```python
from build123d import *

# Parameters (mm, degrees)
BOSS_EXTRUDE1_DEPTH = 3
SKETCH2_R           = 2.125
SKETCH2_R_2         = 1.375
CUT_EXTRUDE1_DEPTH  = 57.401986652


with BuildPart() as part:
    # Sketch1 → Boss-Extrude1 (new body)
    with BuildSketch(Plane(origin=(0, 0, 0), x_dir=(1, 0, 0), z_dir=(0, 1, 0))):
        with BuildLine():
            Line((-31.972318339, 0), (13.027681661, 0))
            ThreePointArc((13.027681661, 0), (28.332991201, -15.30530954), (13.027681661, -30.61061908))
            Line((13.027681661, -30.61061908), (-31.972318339, -30.61061908))
            ThreePointArc((-31.972318339, -30.61061908), (-47.277627879, -15.30530954), (-31.972318339, 0))
        make_face()
    extrude(amount=BOSS_EXTRUDE1_DEPTH)

    # Sketch2 → Cut-Extrude1 (cut, through all)
    with BuildSketch(Plane(origin=(0, 3, 0), x_dir=(1, 0, 0), z_dir=(0, 1, 0))):
        with Locations(Location((-31.972318339, -15.30530954, 0), (0, 0, 270))):
            Circle(SKETCH2_R)
        with Locations(Location((-31.972318339, -5.30530954, 0), (0, 0, 270))):
            Circle(SKETCH2_R_2)
        with Locations(Location((-31.972318339, -25.30530954, 0), (0, 0, 90))):
            Circle(SKETCH2_R_2)
        with Locations(Location((13.027681661, -5.30530954, 0), (0, 0, 90))):
            Circle(SKETCH2_R_2)
        with Locations(Location((13.027681661, -15.30530954, 0), (0, 0, 90))):
            Circle(SKETCH2_R)
        with Locations(Location((13.027681661, -25.30530954, 0), (0, 0, 270))):
            Circle(SKETCH2_R_2)
    extrude(amount=-CUT_EXTRUDE1_DEPTH, mode=Mode.SUBTRACT)


solid = part.part
```
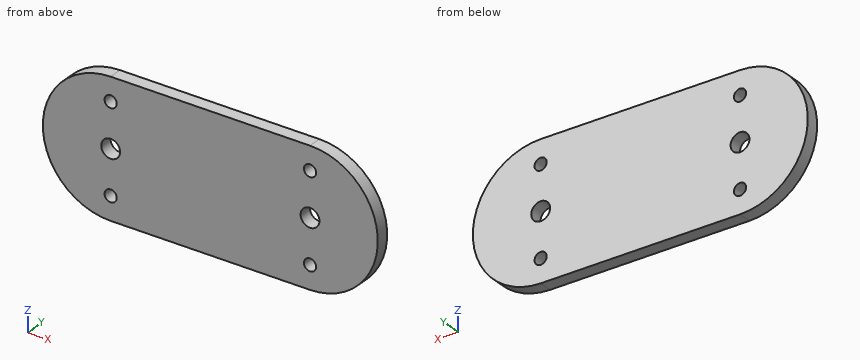
Verification items for the finished model (mm, model axes). Coordinates: 2 decimals unless noted, no trailing zeros. Loops run counter-clockwise (first coordinate to the right, second up) from the corner with the lowest first, then second, coordinate; pieces in that order, holes last. Notation, with made-up numbers: (12.25, 9.25) -> (30.25, 9.25) arc R34 ccw to (30.25, 46.25) -> close; hole circle Ø11 at (0, 11.25). An arc over 180 degrees is marked (long way). Put each result on its own line as item: value.
1. Section check B-B, the plane z = 14. Record the boundary of the cut face in (x, y).
Result set:
outline: (-47.22, 0) -> (-33.65, 0) -> (-33.65, 3) -> (-47.22, 3) -> close; (-30.3, 0) -> (11.35, 0) -> (11.35, 3) -> (-30.3, 3) -> close; (14.7, 0) -> (28.28, 0) -> (28.28, 3) -> (14.7, 3) -> close
2. Section check C-C, the plane z = 8.5. Record the boundary of the cut face in (x, y), then the cut area to 3 significant figures.
Result set:
outline: (-45.68, 0) -> (26.74, 0) -> (26.74, 3) -> (-45.68, 3) -> close
area: 217 mm^2
3. Section check A-A, the plane y = 1.75. Record the boundary of the cut face in (x, z) (3 decimals).
Result set:
outline: (-31.972, 0) -> (13.028, 0) arc R15.305 ccw to (13.028, 30.611) -> (-31.972, 30.611) arc R15.305 ccw to start; hole circle Ø4.25 at (-31.972, 15.305); hole circle Ø2.75 at (-31.972, 5.305); hole circle Ø2.75 at (-31.972, 25.305); hole circle Ø4.25 at (13.028, 15.305); hole circle Ø2.75 at (13.028, 5.305); hole circle Ø2.75 at (13.028, 25.305)
4. Thickness scan on line 1 (Z direction, x = 13, y = 2.4); line 2 (X direction, y = 0.7, z = 25); line 3 (X direction, y = 1.8, z = 14). Record the ranges inside material, lowest first.
Result set:
line 1: z = 0 to 3.93, 6.68 to 13.18, 17.43 to 23.93, 26.68 to 30.61
line 2: x = -43.82 to -33.31, -30.63 to 11.69, 14.37 to 24.87
line 3: x = -47.22 to -33.65, -30.3 to 11.35, 14.7 to 28.28
5. Gauge pin test, flat end, axial feed: P1, Ø5, axis at x = 13.03, z = 15.31, coming from the -Y side. Record the tip position at first contact, or that the pin passes through.
Result set:
P1: stops at y = 0
6. Section check D-D, the plane x = 18. Record the boundary of the cut face in (y, z).
Result set:
outline: (0, 0.83) -> (3, 0.83) -> (3, 29.78) -> (0, 29.78) -> close
